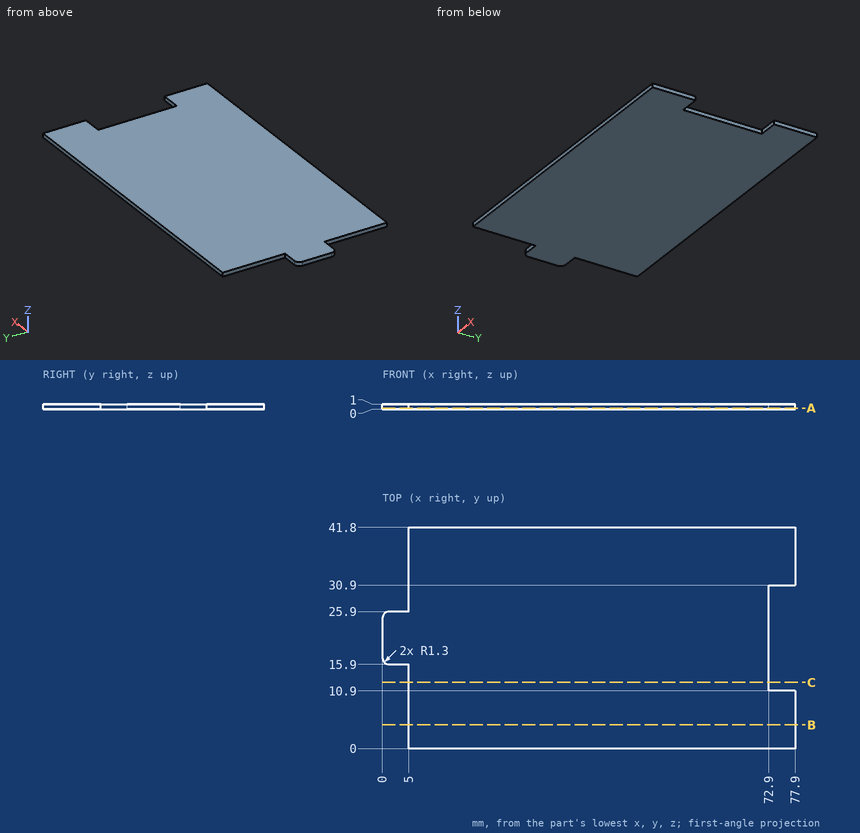
Could you check a few things on this drawing? It's one solid part, dimensions in mm from its lowest x, y, z. Give positions to 0.01 mm unless a question says otherwise; leave off trailing zeros. Order: outer loops, then holes, each group sorted by start corner. A loop starts at its lowest first (then second) coordinate and runs counter-clockwise, first axis right, second up. Notation, with made-up numbers: (19, -21) -> (47, -21) arc R30 cw to (47, 1) -> close; hole circle Ø1 at (84, 80). An arc over 180 degrees is marked (long way). Answer in a Markdown table with one row per item. Add a question column.
Item 1: Please list where these lines run through material, in increasing order: probe 1 along X at (y, z) = (7, 0.75); probe 2 along Y at (x, z) = (75, 0.8); probe 3 along X at (y, z) = (11.5, 0.25).
Item 2: Imagine slicing it at A-A (z = 0.2). List the corners of the cut face in (x, y) for me.
Item 3: Imagine slicing it at B-B (y = 4.5). List the corners of the cut face in (x, z) for me.
Item 4: I'm going to push flat-ended pins straight in: P1, Ø0.5, axis at x = 3.5, z = 0.5, coming from the +Y side; P2, Ø0.5, axis at y = 6.5, z = 0.5, coming from the -X side. Where does each tip first touch, or does it pass through?
Item 5: Imagine slicing it at C-C (y = 12.5). List the corners of the cut face in (x, z) for me.
Result:
| question | item | result |
|---|---|---|
| 1 | probe 1 | 5 to 77.9 |
| 1 | probe 2 | 0 to 10.9, 30.9 to 41.8 |
| 1 | probe 3 | 5 to 72.9 |
| 2 | outline | (0, 17.2) arc R1.3 ccw to (1.3, 15.9) -> (5, 15.9) -> (5, 0) -> (77.9, 0) -> (77.9, 10.9) -> (72.9, 10.9) -> (72.9, 30.9) -> (77.9, 30.9) -> (77.9, 41.8) -> (5, 41.8) -> (5, 25.9) -> (1.3, 25.9) arc R1.3 ccw to (0, 24.6) -> close |
| 3 | outline | (5, 0) -> (77.9, 0) -> (77.9, 1) -> (5, 1) -> close |
| 4 | P1 | y = 25.9 |
| 4 | P2 | x = 5 |
| 5 | outline | (5, 0) -> (72.9, 0) -> (72.9, 1) -> (5, 1) -> close |
